Design review of the part built by this model. Coordinates are the model's own, in mm. Face numbers are marked on the shaded views. A direction names the side the tool comes from. Coordinates: 2 decimals unless noted, no trailing zeros. Order: outer loops, then holes, each group sorted by start corner. A loop starts at its lowest first (then second) coordinate and runs counter-clockwise, first axis right, second up. Notation, with made-up numbers: (31, 13.5) -> (37, 13.5) arc R17 ccw to (37, 28.5) -> close; hole circle Ø2 at (32.5, -36.5). An arc over 180 degrees is marked (long way). Write item = value, one per line.
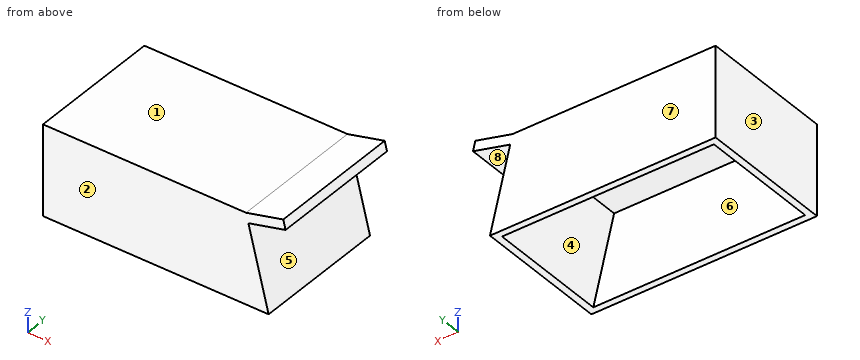
```python
from build123d import *

# Parameters (mm, degrees)
F1_DEPTH = 60
F2_DEPTH = 60
F3_T     = -3


with BuildPart() as f1:
    # F0 (on Front) → F1 (new body)
    with BuildSketch(Plane.XZ):
        Polygon((-57.1974544724, 40), (-57.1974544724, 0), (42.8025455276, 0), (33.833321934, 35.8768943744), (32.8025455276, 40), align=None)
    extrude(amount=F1_DEPTH)

    # F0 (on Front) → F2 (join)
    with BuildSketch(Plane.XZ):
        Polygon((32.8025455276, 40), (33.833321934, 35.8768943744), (50.3257444365, 40), (49.2949680301, 44.1231056256), align=None)
    extrude(amount=F2_DEPTH)

    # F3
    f3_openings = [f1.faces().sort_by_distance(p)[0] for p in [
        (-7.197454, -30, 0),
    ]]
    offset(amount=F3_T, openings=f3_openings, kind=Kind.INTERSECTION)


solid = f1.part
```
(1) For L1, parallel to Y at x = -15.5, z = 11; L2, parallel to X at y = -49.5, z = 5; L3, parallel to X at y = -56, z = 30, list the stretches that pass through material, from the lowest coordinate up.
Report:
L1 = -60 to -57, -3 to 0
L2 = -57.2 to -54.2, 38.46 to 41.55
L3 = -57.2 to -54.2, 32.21 to 35.3
(2) We need section D-D (z = 13). Write out the cut boundary in (x, y), and give its area (3 significant figures).
Report:
outline = (-57.2, -60) -> (39.55, -60) -> (39.55, 0) -> (-57.2, 0) -> close; hole (-54.2, -57) -> (36.46, -57) -> (36.46, -3) -> (-54.2, -3) -> close
area = 909 mm²
(3) For the marked faces 1, 2, 3, 4 and 5, list the 3-axis set-ups (+Z, -Z, +X, -X, +Y, -Y) from which the entire face can be reached by the end or side of a thin tool; tool diameter is ignored.
Report:
face_1 = +Z, -X, +Y, -Y
face_2 = +Z, -Z, +X, -X, -Y
face_3 = +Z, -Z, -X, +Y, -Y
face_4 = -Z
face_5 = +X, +Y, -Y
(4) Insertion check: pin 1 (5 mm diameter, centred on x = -45.5, y = -53.5, fed in from +Z); pin 2 (8 mm diameter, centred on x = -32, y = -46.5, fed in from -Z); pin 3 (3 mm diameter, centred on y = -14, z = 4.5, fed in from +X). Each pin has a flat end and moves straight along its axis. Give the tip position at first contact, or say it passes through.
Report:
pin_1 = 40
pin_2 = 37
pin_3 = 42.05
(5) We need section A-A (y = -26). Write out the cut boundary in (x, z).
Report:
outline = (-57.2, 0) -> (-54.2, 0) -> (-54.2, 37) -> (30.46, 37) -> (39.71, 0) -> (42.8, 0) -> (33.83, 35.88) -> (50.33, 40) -> (49.29, 44.12) -> (32.8, 40) -> (-57.2, 40) -> close
(6) We need section B-B (z = 7). Write out the cut boundary in (x, y).
Report:
outline = (-57.2, -60) -> (41.05, -60) -> (41.05, 0) -> (-57.2, 0) -> close; hole (-54.2, -57) -> (37.96, -57) -> (37.96, -3) -> (-54.2, -3) -> close
(7) We need section C-C (x = 2). Write out the cut boundary in (y, z), and give its area (3 significant figures).
Report:
outline = (-60, 0) -> (-57, 0) -> (-57, 37) -> (-3, 37) -> (-3, 0) -> (0, 0) -> (0, 40) -> (-60, 40) -> close
area = 402 mm²
(8) The part is to be moulded in two halves that separate along X. For the marked faces 6, 7 and 8, say which applies: released by +X, released by -X, zero draft, split by the parting line, or undercut.
Report:
face_6 = undercut
face_7 = zero draft
face_8 = released by +X
